from build123d import *

# Parameters (mm, degrees)
SKETCH1_W           = 3.58775
SKETCH1_H           = 3.175
BOSS_EXTRUDE1_DEPTH = 3.175


with BuildPart() as part:
    # Sketch1 → Boss-Extrude1 (new body)
    with BuildSketch(Plane.XY):
        with BuildLine():
            Line((0, 3.7465), (0, 0))
            Line((0, 0), (12.7, 0))
            Line((12.7, 0), (19.05, 25.4))
            Line((19.05, 25.4), (11.46175, 25.4))
            Line((11.46175, 25.4), (11.46175, 17.526))
            Line((11.46175, 17.526), (13.49375, 17.526))
            Line((13.49375, 17.526), (13.49375, 14.986))
            Line((13.49375, 14.986), (11.46175, 14.986))
            Line((11.46175, 14.986), (11.46175, 9.652))
            Line((11.46175, 9.652), (8.66775, 9.652))
            Line((8.66775, 9.652), (8.66775, 14.986))
            Line((8.66775, 14.986), (6.63575, 14.986))
            Line((6.63575, 14.986), (6.63575, 17.526))
            Line((6.63575, 17.526), (8.66775, 17.526))
            Line((8.66775, 17.526), (8.66775, 25.4))
            Line((8.66775, 25.4), (3.58775, 25.4))
            Line((3.58775, 25.4), (0, 25.4))
            Line((0, 25.4), (0, 6.4135))
            ThreePointArc((0, 6.4135), (0.942926893, 6.022926893), (1.3335, 5.08))
            ThreePointArc((1.3335, 5.08), (0.942926893, 4.137073107), (0, 3.7465))
        make_face()
        with BuildLine():
            Line((-12.7, 0), (0, 0))
            Line((0, 0), (0, 3.7465))
            ThreePointArc((0, 3.7465), (-1.3335, 5.08), (0, 6.4135))
            Line((0, 6.4135), (0, 25.4))
            Line((0, 25.4), (-3.58775, 25.4))
            Line((-3.58775, 25.4), (-8.66775, 25.4))
            Line((-8.66775, 25.4), (-8.66775, 17.526))
            Line((-8.66775, 17.526), (-6.63575, 17.526))
            Line((-6.63575, 17.526), (-6.63575, 14.986))
            Line((-6.63575, 14.986), (-8.66775, 14.986))
            Line((-8.66775, 14.986), (-8.66775, 9.652))
            Line((-8.66775, 9.652), (-10.06475, 9.652))
            Line((-10.06475, 9.652), (-11.46175, 9.652))
            Line((-11.46175, 9.652), (-11.46175, 14.986))
            Line((-11.46175, 14.986), (-13.49375, 14.986))
            Line((-13.49375, 14.986), (-13.49375, 17.526))
            Line((-13.49375, 17.526), (-11.46175, 17.526))
            Line((-11.46175, 17.526), (-11.46175, 25.4))
            Line((-11.46175, 25.4), (-19.05, 25.4))
            Line((-19.05, 25.4), (-12.7, 0))
        make_face()
        with Locations((1.793875, 26.9875)):
            Rectangle(SKETCH1_W, SKETCH1_H)
        with Locations((-1.793875, 26.9875)):
            Rectangle(SKETCH1_W, SKETCH1_H)
    extrude(amount=BOSS_EXTRUDE1_DEPTH)


solid = part.part
CAD build for the part. Positions are in the model's coordinates, mm. A direction names the side the tool comes from. Coordinates: 2 decimals unless noted, no trailing zeros. Order: outer loops, then holes, each group sorted by start corner. A loop starts at its lowest first (then second) coordinate and runs counter-clockwise, first axis right, second up. Notation, with made-up numbers: (70, 76.5) -> (124, 76.5) arc R27 cw to (124, 114.5) -> close; hole circle Ø11 at (72, 34). An arc over 180 degrees is marked (long way). Answer in a Markdown table with one row per item.
1) Flat gauge pins, fed straight in: P1, Ø1.4, axis at x = 10.5, z = 1, coming from the +Y side; P2, Ø1.6, axis at y = 27, z = 1.5, coming from the +X side; P3, Ø1.6, axis at x = -14.5, z = 1, coming from the +Y side. Where does each tip first touch, or does it go through?
Check values:
| item | result |
|---|---|
| P1 | y = 9.65 |
| P2 | x = 3.59 |
| P3 | y = 25.4 |
2) Band-saw the part on B-B (y = 23.75). List the corners of the cut face in (x, z) (1 decimal), and give its area (3 significant figures).
Check values:
| item | result |
|---|---|
| outline | (-18.6, 0) -> (-11.5, 0) -> (-11.5, 3.2) -> (-18.6, 3.2) -> close; (-8.7, 0) -> (8.7, 0) -> (8.7, 3.2) -> (-8.7, 3.2) -> close; (11.5, 0) -> (18.6, 0) -> (18.6, 3.2) -> (11.5, 3.2) -> close |
| area | 101 mm2 |
3) Which spindle directions (+Z, -Z, +X, -X, +Y, -Y) get a long thin tool onto all of the face, cutting with end or side? Do faces 1 (the face through (-3.588, 27, 2)), 2 (the face through (11.462, 22, 2)), 3 (the face through (12, 17.526, 2)). Say none if no direction does.
Check values:
| item | result |
|---|---|
| face 1 | +Z, -Z, -X, +Y |
| face 2 | +Z, -Z, +Y |
| face 3 | +Z, -Z |
4) Drill centre lines: line 1 (X direction, y = 11.25, z = 1.45); line 2 (Y direction, x = -12, z = 0.7); line 3 (X direction, y = 12.75, z = 2.15). Where is each one in solid material? Low to high.
Check values:
| item | result |
|---|---|
| line 1 | -15.51 to -11.46, -8.67 to 8.67, 11.46 to 15.51 |
| line 2 | 0 to 14.99, 17.53 to 25.4 |
| line 3 | -15.89 to -11.46, -8.67 to 8.67, 11.46 to 15.89 |
5) Band-saw the part on A-A (y = 12). List the corners of the cut face in (x, z) (3 decimals), and give its area (3 significant figures).
Check values:
| item | result |
|---|---|
| outline | (-15.7, 0) -> (-11.462, 0) -> (-11.462, 3.175) -> (-15.7, 3.175) -> close; (-8.668, 0) -> (8.668, 0) -> (8.668, 3.175) -> (-8.668, 3.175) -> close; (11.462, 0) -> (15.7, 0) -> (15.7, 3.175) -> (11.462, 3.175) -> close |
| area | 82.0 mm2 |
6) Band-saw the part on D-D (x = 4.5). List the corners of the cut face in (y, z) (3 decimals), and give its area (3 significant figures).
Check values:
| item | result |
|---|---|
| outline | (0, 0) -> (25.4, 0) -> (25.4, 3.175) -> (0, 3.175) -> close |
| area | 80.6 mm2 |
7) Mould opens along Y. For faces 4 (the face through (0, 0, 2)), 5 (the face through (8, 14.986, 2)), 6 (the face through (-11.462, 12, 2)) say: pulls with the +Y half, pulls with the -Y half, needs draft (parallel to the pull), parting line crosses it, or undercut.
Check values:
| item | result |
|---|---|
| face 4 | pulls with the -Y half |
| face 5 | undercut |
| face 6 | needs draft |
8) Band-saw the part on C-C (x = 11). List the corners of the cut face in (y, z) (3 decimals), and give its area (3 significant figures).
Check values:
| item | result |
|---|---|
| outline | (0, 0) -> (9.652, 0) -> (9.652, 3.175) -> (0, 3.175) -> close |
| area | 30.6 mm2 |
